Autodesk Inventor part; units mm, degrees
ref_plane "YZ Plane" through (0, 0, 0) normal (1, 0, 0) x (0, 1, 0)
ref_plane "XZ Plane" through (0, 0, 0) normal (0, 1, 0) x (-1, 0, 0)
ref_plane "XY Plane" through (0, 0, 0) normal (0, 0, 1) x (1, 0, 0)
sketch "Sketch1" plane through (0, 0, 0) normal (0, 1, 0) x (-1, 0, 0)
  line L0 (0, 0) -> (15, 0)
  line L1 (15, 0) -> (15, -110)
  line L2 (15, -110) -> (0, -110)
  line L3 (0, -110) -> (0, 0)
  dimension "d0" = 110
  dimension "d1" = 15
extrude "Extrusion1" add sketch "Sketch1" along normal blind 10
sketch "Sketch2" plane through (0, 10, 0) normal (0, 1, 0) x (1, 0, 0)
  line L0 (-15, 0) -> (0, 0)
  line L1 (0, 0) -> (0, 110)
  line L2 (-15, 0) -> (0, 0)
  line L3 (0, 0) -> (0, 10)
  line L4 (0, 10) -> (-15, 10)
  line L5 (-15, 10) -> (-15, 0)
  line L6 (0, 110) -> (-15, 110)
  line L7 (-15, 110) -> (0, 110)
  line L8 (0, 110) -> (0, 100)
  line L9 (0, 100) -> (-15, 100)
  line L10 (-15, 100) -> (-15, 110)
  dimension "d4" = 10
  dimension "d5" = 10
extrude "Extrusion2" add sketch "Sketch2" along normal blind 18
sketch "Sketch3" plane through (0, 28, 0) normal (0, 1, 0) x (1, 0, 0)
  line L0 (0, 0) -> (0, 10)
  line L1 (0, 10) -> (-50, 10)
  line L2 (-50, 10) -> (-50, -10)
  line L3 (-50, -10) -> (0, -10)
  line L4 (0, -10) -> (0, 10)
  line L5 (-15, 100) -> (0, 100)
  line L6 (0, 100) -> (-50, 100)
  line L7 (-50, 100) -> (-50, 120)
  line L8 (-50, 120) -> (0, 120)
  line L9 (0, 120) -> (0, 100)
  dimension "d8" = 50
  dimension "d9" = 20
  dimension "d10" = 50
  dimension "d11" = 20
extrude "Extrusion3" add sketch "Sketch3" along normal blind 2
properties part number "servobridge"
The listing builds one solid part. Answer for the finished solid, in the listing's coordinates (mm). A direction names the side the tool comes from. Coordinates: 2 decimals unless noted, no trailing zeros. Write each loop counter-clockwise with the first axis right and the second up, starting at its lowest first coordinate (ties: lowest second). Pieces come first, ordered by that corner, then holes.
Q1. Section D-D, the plane z = -88 is taken. Write down the section's boundary in (x, y).
Returned:
outline: (-15, 0) - (0, 0) - (0, 10) - (-15, 10) - close
Q2. Given P1, Ø4.5, axis at x = -6, y = 19.5, coming from the +Z side; P2, Ø10, axis at x = -31.5, z = 3.5, coming from the -Y side; P3, Ø14, axis at y = 7.5, z = -79, coming from the -X side, each flat-ended and moving along its own axis, determine where each tip first touches the part or whether it passes through.
Returned:
P1: stops at z = 0
P2: stops at y = 28
P3: stops at x = -15
Q3. Section A-A, the plane y = 23 is taken. Write down the section's boundary in (x, z), then the cut area to 3 significant figures.
Returned:
outline: (-15, -110) - (0, -110) - (0, -100) - (-15, -100) - close; (-15, -10) - (0, -10) - (0, 0) - (-15, 0) - close
area: 300 mm2
Q4. Which of the six approach directions +Z, -Z, +X, -X, +Y, -Y give full straight-line access (tool end or side, diameter ignored) to faces 5 (the flat face through (-7, 10, -54)), 6 (the flat face through (-7, 0, -54))?
Returned:
face 5: +X, -X, +Y
face 6: +Z, -Z, +X, -X, -Y
Q5. Find the intervals of material crossed by line 1 along X through (y, z) = (15.5, -105); line 2 along Y through (x, z) = (-19.5, 2.5); line 3 along Y through (x, z) = (-12, -71), in increasing order.
Returned:
line 1: x = -15 to 0
line 2: y = 28 to 30
line 3: y = 0 to 10
Q6. Section C-C, the plane x = -4 is taken. Write down the section's boundary in (y, z), then the cut area to 3 significant figures.
Returned:
outline: (0, -110) - (28, -110) - (28, -120) - (30, -120) - (30, -100) - (10, -100) - (10, -10) - (30, -10) - (30, 10) - (28, 10) - (28, 0) - (0, 0) - close
area: 1,540 mm2
Q7. Section B-B, the plane x = -44 is taken. Write down the section's boundary in (y, z), then the cut area to 3 significant figures.
Returned:
outline: (28, -120) - (30, -120) - (30, -100) - (28, -100) - close; (28, -10) - (30, -10) - (30, 10) - (28, 10) - close
area: 80.0 mm2
Q8. The mould has two halves that part along Z. Classify faces 1 (the flat face through (-14, 22, -10)), 2 (the flat face through (-7, 14, 0)), 3 (the flat face through (-8, 14, -110)), 4 (the flat face through (-15, 8, -54)): released by +Z, released by -Z, zero draft, split by the parting line, or undercut.
Returned:
face 1: undercut
face 2: released by +Z
face 3: released by -Z
face 4: zero draft
